Source: CAD feature listing. Evaluate the final solid. Frame: model axes, mm. A direction names the side the tool comes from. Coordinates: 2 decimals unless noted, no trailing zeros. Order: outer loops, then holes, each group sorted by start corner. A loop starts at its lowest first (then second) coordinate and runs counter-clockwise, first axis right, second up. Notation, with made-up numbers: (88.5, 9.5) -> (121.5, 9.5) arc R28 ccw to (121.5, 43.5) -> close; hole circle Ø10 at (-30.5, 20). An arc over 180 degrees is marked (long way). Write each question's results on one line, items separated by ' | '. Start each with the question number.
from build123d import *

# Parameters (mm, degrees)
SKETCH1_R           = 10
BOSS_EXTRUDE1_DEPTH = 18
SKETCH2_R           = 10
SKETCH2_R_2         = 4
BOSS_EXTRUDE2_DEPTH = 5


with BuildPart() as part:
    # Sketch1 → Boss-Extrude1 (new body)
    with BuildSketch(Plane.XY):
        Circle(SKETCH1_R)
        with BuildLine():
            Line((-6.5, 3.741657387), (-6.5, -3.741657387))
            ThreePointArc((-6.5, -3.741657387), (0, -7.5), (6.5, -3.741657387))
            Line((6.5, -3.741657387), (6.5, 3.741657387))
            ThreePointArc((6.5, 3.741657387), (0, 7.5), (-6.5, 3.741657387))
        make_face(mode=Mode.SUBTRACT)
    extrude(amount=BOSS_EXTRUDE1_DEPTH)

    # Sketch2 → Boss-Extrude2 (add)
    with BuildSketch(Plane(origin=(0, 0, 0), x_dir=(-1, 0, 0), z_dir=(0, 0, -1))):
        Circle(SKETCH2_R)
        Circle(SKETCH2_R_2, mode=Mode.SUBTRACT)
    extrude(amount=BOSS_EXTRUDE2_DEPTH)


solid = part.part
(1) Section D-D on y = -0.5. Return the cut outline in (x, z).
(2) First-contact query: P1, Ø4, axis at x = 3.5, y = 0.5, coming from the -Z side; P2, Ø2, axis at y = -1.5, z = 11.5, coming from the +X side; P3, Ø7, axis at x = 0, y = 0, coming from the +Z side; P4, Ø10, axis at y = -6, z = 3, coming from the -X side. Flat tips, straight axial feed; report the tip coordinate or a pass-through.
(3) Draft query along X for faces 3 (the flat face through (0.1, -4.3, -5)), 4 (the cylindrical face through (-0.1, -7.5, 8.9)). Return one class per face: released by +X, released by -X, zero draft, split by the parting line, or undercut.
(4) Section C-C on y = -6. Return the cut outline in (x, z).
(5) Line query: L1, parallel to Y at x = 0, z = -3.8; L2, parallel to Z at x = -0.5, y = 5; L3, parallel to Y at x = -2.75, z = 4.5. Output: solid intervals per line, ascending.
(6) Section B-B on z = 10.75. Return the cut outline in (x, y), then the cut area to 3 significant figures.
(7) Section A-A on x = 0. Return the cut outline in (y, z), then the cut area to 3 significant figures.
(8) Reachability of faces 1 (the flat face through (-6.5, 0, 9)), 2 (the flat face through (7, 0, 18)) from +Z, -Z, +X, -X, +Y, -Y: full face, straight path, thin tool, end or side. Return the list, or none.
Results list:
1) outline: (-9.99, -5) -> (-3.97, -5) -> (-3.97, 0) -> (-6.5, 0) -> (-6.5, 18) -> (-9.99, 18) -> close; (3.97, -5) -> (9.99, -5) -> (9.99, 18) -> (6.5, 18) -> (6.5, 0) -> (3.97, 0) -> close
2) P1: stops at z = -5 | P2: stops at x = 9.99 | P3: passes through | P4: stops at x = -9.95
3) face 3: zero draft | face 4: undercut
4) outline: (-8, -5) -> (8, -5) -> (8, 18) -> (4.5, 18) -> (4.5, 0) -> (-4.5, 0) -> (-4.5, 18) -> (-8, 18) -> close
5) L1: y = -10 to -4, 4 to 10 | L2: z = -5 to 0 | L3: y = -9.61 to -6.98, 6.98 to 9.61
6) outline: circle Ø20 at (0, 0); hole (-6.5, -3.74) arc R7.5 ccw to (6.5, -3.74) -> (6.5, 3.74) arc R7.5 ccw to (-6.5, 3.74) -> close | area: 148 mm²
7) outline: (-10, -5) -> (-4, -5) -> (-4, 0) -> (-7.5, 0) -> (-7.5, 18) -> (-10, 18) -> close; (4, -5) -> (10, -5) -> (10, 18) -> (7.5, 18) -> (7.5, 0) -> (4, 0) -> close | area: 150 mm²
8) face 1: +Z | face 2: +Z, +X, -X, +Y, -Y
